Design review of the part shown in the three views and the two pictorial views. Dimensions are in mm from the part's minimum x, y and z. Coordinates: 2 decimals unless noted, no trailing zeros. Loops run counter-clockwise (first coordinate to the right, second up) from the corner with the lowest first, then second, coordinate; pieces in that order, holes last.
Q1. Add section B-B on z = 1.8. Give the boundary of the cut face in (x, y).
Q2. Wall thickness on probe 1 along Y at (x, z) = (9, 0.85); probe 2 along X at (y, z) = (28, 0.35); probe 3 along Y at (x, z) = (6.75, 2.05): over which ranges is each line inside the solid? List them lowest first.
Q3. Add section D-D on x = 19.25. Give the boundary of the cut face in (y, z).
Q4. Add section A-A on x = 16.75. Give the boundary of the cut face in (y, z).
Q5. For P1, Ø1.4, axis at x = 15.5, y = 42, coming from the +Z side; P2, Ø1, axis at x = 3.5, y = 25, coming from the -Z side; P3, Ø1, axis at x = 3.5, y = 14.5, coming from the -Z side; P4, Ø1, axis at y = 15, z = 0.5, coming from the -X side, all flat-tipped, find the tip position at first contact; note any pin that passes through.
Q6. Add section C-C on x = 11.5. Give the boundary of the cut face in (y, z).
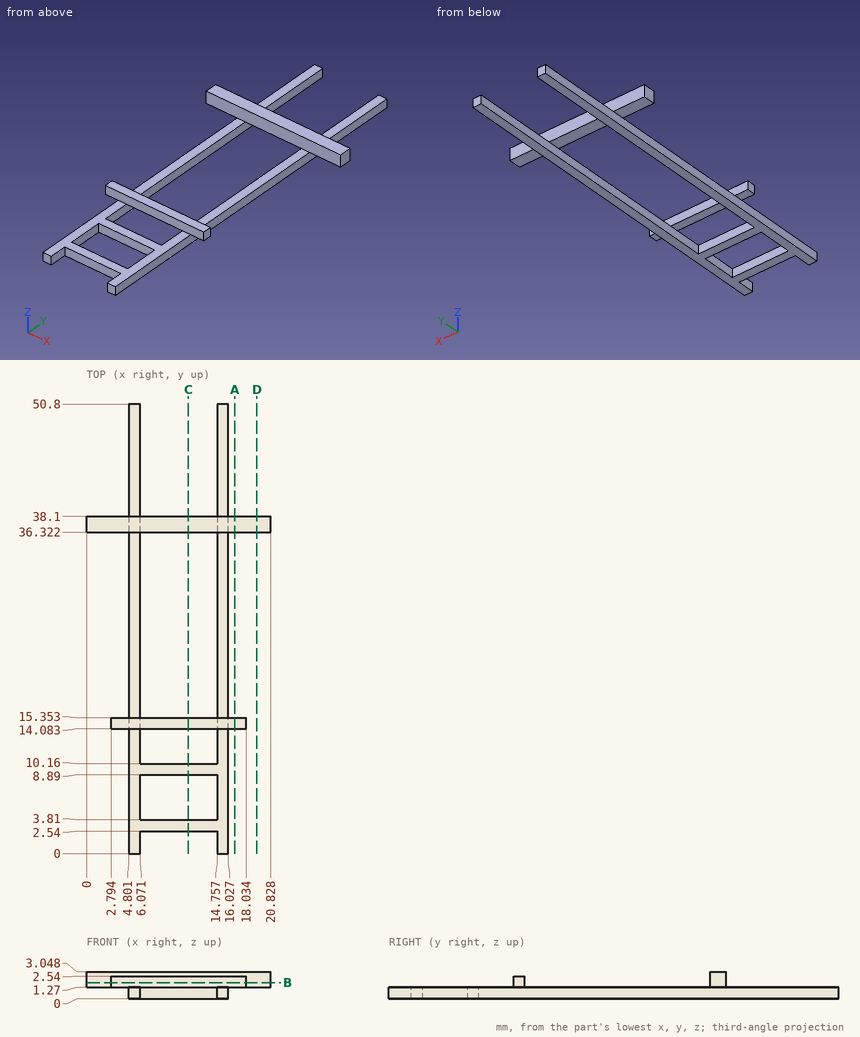
Entries:
1. outline: (0, 36.32) - (20.83, 36.32) - (20.83, 38.1) - (0, 38.1) - close; (2.79, 14.08) - (18.03, 14.08) - (18.03, 15.35) - (2.79, 15.35) - close
2. probe 1: y = 2.54 to 3.81, 8.89 to 10.16
2. probe 2: x = 4.8 to 6.07, 14.76 to 16.03
2. probe 3: y = 14.08 to 15.35, 36.32 to 38.1
3. outline: (36.32, 1.27) - (38.1, 1.27) - (38.1, 3.05) - (36.32, 3.05) - close
4. outline: (14.08, 1.27) - (15.35, 1.27) - (15.35, 2.54) - (14.08, 2.54) - close; (36.32, 1.27) - (38.1, 1.27) - (38.1, 3.05) - (36.32, 3.05) - close
5. P1: stops at z = 1.27
5. P2: passes through
5. P3: stops at z = 1.27
5. P4: stops at x = 4.8
6. outline: (2.54, 0) - (3.81, 0) - (3.81, 1.27) - (2.54, 1.27) - close; (8.89, 0) - (10.16, 0) - (10.16, 1.27) - (8.89, 1.27) - close; (14.08, 1.27) - (15.35, 1.27) - (15.35, 2.54) - (14.08, 2.54) - close; (36.32, 1.27) - (38.1, 1.27) - (38.1, 3.05) - (36.32, 3.05) - close
